Verification items for this drawing (mm, ordinates from the low corner). Round coordinates to 2 decimals unless told otherwise and drop trailing zeros. Loops run counter-clockwise (first coordinate to the right, second up) from the corner with the lowest first, then second, coordinate; pieces in that order, holes last. Notation, with made-up numbers: M -35.75,30 L -7.75,30 A15 cw -7.75,37 Z; hole C 78.5,6 d5. An arc over 180 degrees is marked long. Write item = value, one per line. Start each with the question number.
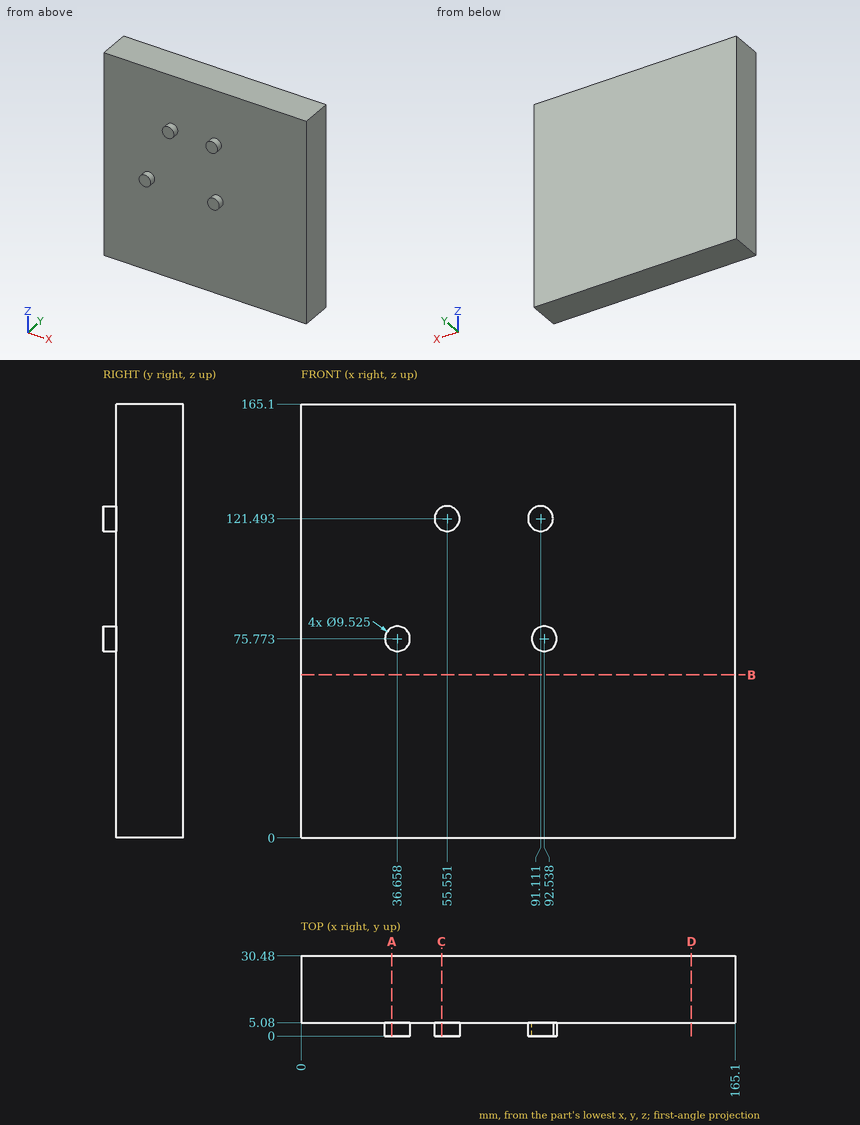
1. Thickness scan on line 1 (Y direction, x = 87, z = 102). Record the ranges inside material, lowest first.
2. Section check A-A, the plane x = 34.5. Enter the section's corners in (y, z), and give its area (3 significant figures).
3. Section check C-C, the plane x = 53.5. Enter the section's corners in (y, z) (1 decimal).
4. Section check B-B, the plane z = 62. Enter the section's corners in (x, y).
5. Section check D-D, the plane x = 148.5. Enter the section's corners in (y, z), and give its area (3 significant figures).
Computed values:
q1.line_1 = 5.08 to 30.48
q2.outline = M 0,71.53 L 5.08,71.53 L 5.08,0 L 30.48,0 L 30.48,165.1 L 5.08,165.1 L 5.08,80.02 L 0,80.02 Z
q2.area = 4,240 mm2
q3.outline = M 0,117.2 L 5.1,117.2 L 5.1,0 L 30.5,0 L 30.5,165.1 L 5.1,165.1 L 5.1,125.8 L 0,125.8 Z
q4.outline = M 0,5.08 L 165.1,5.08 L 165.1,30.48 L 0,30.48 Z
q5.outline = M 5.08,0 L 30.48,0 L 30.48,165.1 L 5.08,165.1 Z
q5.area = 4,190 mm2
